from build123d import *

# Parameters (mm, degrees)
SKETCH_1_W      = 35.928
SKETCH_1_H      = 35.088
EXTRUDE_2_DEPTH = 1
SKETCH_1_5_W    = 71.856
SKETCH_1_5_H    = 70.176
EXTRUDE_5_DEPTH = 3.4
EXTRUDE_6_DEPTH = 3.41


with BuildPart() as part:
    # Sketch 1 → Extrude 2 (new body)
    with BuildSketch(Plane.XY):
        Polygon((0, 38.09), (0, 35.088), (35.928, 35.088), (35.928, 0), (37.13, 0), (37.13, 38.09), align=None)
        Polygon((-41.5, 0), (-37.13, 0), (-37.13, 38.09), (0, 38.09), (0, 41.5), (-41.5, 41.5), align=None)
        Polygon((-37.13, 0), (-35.928, 0), (-35.928, 35.088), (0, 35.088), (0, 38.09), (-37.13, 38.09), align=None)
        Polygon((0, 41.5), (0, 38.09), (37.13, 38.09), (37.13, 0), (41.5, 0), (41.5, 41.5), align=None)
        with Locations((17.964, 17.544)):
            Rectangle(SKETCH_1_W, SKETCH_1_H)
        with Locations((-17.964, 17.544)):
            Rectangle(SKETCH_1_W, SKETCH_1_H)
        with Locations((-17.964, -17.544)):
            Rectangle(SKETCH_1_W, SKETCH_1_H)
        with Locations((17.964, -17.544)):
            Rectangle(SKETCH_1_W, SKETCH_1_H)
        Polygon((37.13, -38.09), (0, -38.09), (0, -41.5), (41.5, -41.5), (41.5, 0), (37.13, 0), align=None)
        Polygon((35.928, -35.088), (0, -35.088), (0, -38.09), (37.13, -38.09), (37.13, 0), (35.928, 0), align=None)
        Polygon((0, -35.088), (-35.928, -35.088), (-35.928, 0), (-37.13, 0), (-37.13, -38.09), (0, -38.09), align=None)
        Polygon((-37.13, -38.09), (-37.13, 0), (-41.5, 0), (-41.5, -41.5), (0, -41.5), (0, -38.09), align=None)
    extrude(amount=EXTRUDE_2_DEPTH)

    # Sketch 1_5 → Extrude 5 (add)
    with BuildSketch(Plane.XY):
        Rectangle(SKETCH_1_5_W, SKETCH_1_5_H)
    extrude(amount=EXTRUDE_5_DEPTH)

    # Sketch 1_6 → Extrude 6 (add)
    with BuildSketch(Plane.XY):
        Polygon((-37.13, 0), (-35.928, 0), (-35.928, 35.088), (0, 35.088), (0, 38.09), (-37.13, 38.09), align=None)
        Polygon((0, 38.09), (0, 35.088), (35.928, 35.088), (35.928, 0), (37.13, 0), (37.13, 38.09), align=None)
        Polygon((35.928, -35.088), (0, -35.088), (0, -38.09), (37.13, -38.09), (37.13, 0), (35.928, 0), align=None)
        Polygon((0, -35.088), (-35.928, -35.088), (-35.928, 0), (-37.13, 0), (-37.13, -38.09), (0, -38.09), align=None)
    extrude(amount=EXTRUDE_6_DEPTH)


solid = part.part
Input: part model. Units: mm. Frame: model coordinates. A direction names the side the tool comes from. Give positions to 0.01 mm unless a question says otherwise; leave off trailing zeros. Write each loop counter-clockwise with the first axis right and the second up, starting at its lowest first coordinate (ties: lowest second). Pieces come first, ordered by that corner, then holes.
Q1. Section C-C, the plane z = 2.1. Output: boundary loops of the cut face in (x, y).
Q2. Material intervals for probe 1 along Y at (x, z) = (17, 1.05); probe 2 along Z at (x, y) = (35.5, -29.5); probe 3 along X at (y, z) = (21.5, 3.05), sorted ascending.
Q3. First-contact query: P1, Ø0.7, axis at x = -8.5, z = 1.5, coming from the +Y side; P2, Ø1.2, axis at x = 11.5, z = 2.5, coming from the -Y side; P3, Ø1, axis at y = -27.5, z = 2.5, coming from the +X side. Flat tips, straight axial feed; report the tip coordinate or a pass-through.
Q4. Set-up query: faces 1 (the face through (1, 38.09, 2)), 2 (the face through (37.13, -1, 2)), 3 (the face through (-1, -38.09, 2)). Return all of +Z, -Z, +X, -X, +Y, -Y with unobstructed straight access to the full face (end or side cutting, diameter ignored); none if empty.
Filled in:
1. outline: (-37.13, -38.09) - (37.13, -38.09) - (37.13, 38.09) - (-37.13, 38.09) - close
2. probe 1: y = -38.09 to 38.09
2. probe 2: z = 0 to 3.4
2. probe 3: x = -37.13 to 37.13
3. P1: stops at y = 38.09
3. P2: stops at y = -38.09
3. P3: stops at x = 37.13
4. face 1: +Z, +X, -X, +Y
4. face 2: +Z, +X, +Y, -Y
4. face 3: +Z, +X, -X, -Y
